The listing builds one solid part. Answer for the finished solid, in the listing's coordinates (mm). Face numbers are marked on the shaded views. A direction names the side the tool comes from. Give positions to 0.01 mm unless a question says otherwise; leave off trailing zeros. Order: outer loops, then holes, each group sorted by start corner. A loop starts at its lowest first (then second) coordinate and runs counter-clockwise, first axis right, second up.
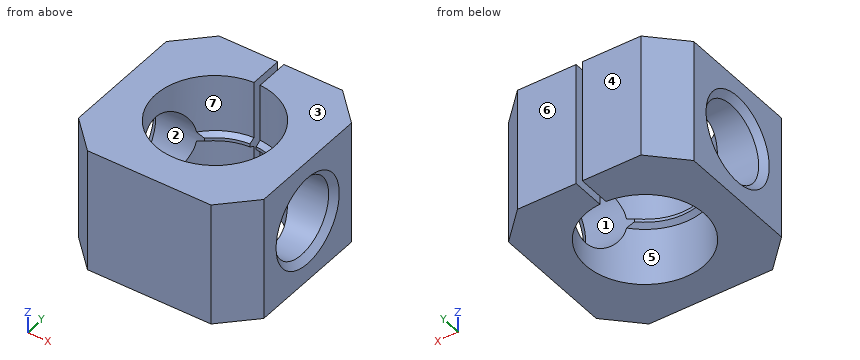
```python
from build123d import *

# Parameters (mm, degrees)
SKETCH047_W     = 30
SKETCH047_H     = 30
SKETCH047_R     = 9.6
PAD018_DEPTH    = 20
SKETCH049_W     = 1
SKETCH049_H     = 15
POCKET028_DEPTH = 20
SKETCH050_R     = 6.2
POCKET029_DEPTH = 40
CHAMFER004_SIZE = 1
CHAMFER005_SIZE = 5


with BuildPart() as part:
    # Sketch047 → Pad018 (new body)
    with BuildSketch(Plane.XY):
        Rectangle(SKETCH047_W, SKETCH047_H)
        Circle(SKETCH047_R, mode=Mode.SUBTRACT)
    extrude(amount=PAD018_DEPTH)

    # Sketch048 → Revolution002 (revolve)
    with BuildSketch(Plane.YZ):
        Polygon((9.6, 10.75), (9.6, 9.25), (8.7, 9.75), (8.7, 10.25), align=None)
    revolve(axis=Axis((0, 0, 0), (0, 0, 1)))

    # Sketch049 (on Face11 of Revolution002) → Pocket028 (cut)
    with BuildSketch(Plane.XY.offset(20)):
        with Locations((0, 7.5)):
            Rectangle(SKETCH049_W, SKETCH049_H)
    extrude(amount=-POCKET028_DEPTH, mode=Mode.SUBTRACT)

    # Sketch050 (on Face12 of Pocket028) → Pocket029 (cut)
    with BuildSketch(Plane(origin=(-15, 0, 0), x_dir=(0, -1, 0), z_dir=(-1, 0, 0))):
        with Locations((0, 10)):
            Circle(SKETCH050_R)
    extrude(amount=-POCKET029_DEPTH, mode=Mode.SUBTRACT)

    # Chamfer004
    chamfer004_edges = [part.edges().sort_by_distance(p)[0] for p in [
        (-15, 6.2, 10),
        (15, 6.2, 10),
    ]]
    chamfer(chamfer004_edges, length=CHAMFER004_SIZE)

    # Chamfer005
    chamfer005_edges = [part.edges().sort_by_distance(p)[0] for p in [
        (-15, -15, 10),
        (-15, 15, 10),
        (15, -15, 10),
        (15, 15, 10),
    ]]
    chamfer(chamfer005_edges, length=CHAMFER005_SIZE)


solid = part.part
```
1) Find section B-B (y = 12.5). Write down the section's boundary in (x, z).
Geometry says:
outline: (-12.5, 0) - (-0.5, 0) - (-0.5, 20) - (-12.5, 20) - close; (0.5, 0) - (12.5, 0) - (12.5, 20) - (0.5, 20) - close
2) Find section D-D (z = 17.75). Write down the section's boundary in (x, y).
Geometry says:
outline: (-15, -10) - (-10, -15) - (10, -15) - (15, -10) - (15, 10) - (10, 15) - (0.5, 15) - (0.5, 9.59) arc R9.6 cw (long way) to (-0.5, 9.59) - (-0.5, 15) - (-10, 15) - (-15, 10) - close
3) Find section A-A (y = 0). Write down the section's boundary in (x, z), then the cut area to 3 significant figures.
Geometry says:
outline: (-15, 0) - (-9.6, 0) - (-9.6, 3.8) - (-14, 3.8) - (-15, 2.8) - close; (-15, 17.2) - (-14, 16.2) - (-9.6, 16.2) - (-9.6, 20) - (-15, 20) - close; (9.6, 0) - (15, 0) - (15, 2.8) - (14, 3.8) - (9.6, 3.8) - close; (9.6, 16.2) - (14, 16.2) - (15, 17.2) - (15, 20) - (9.6, 20) - close
area: 80.1 mm2
4) Straight lines are drawn through the part: probe 1 along Z at (x, y) = (-11.25, 0); probe 2 along Y at (x, z) = (-7.5, 10); probe 3 along Y at (x, z) = (-0.25, 18). For each, find the intervals that lie inside material, in ascending order.
Geometry says:
probe 1: z = 0 to 3.8, 16.2 to 20
probe 2: y = -15 to -6.2, 6.2 to 15
probe 3: y = -15 to -9.6
5) Given P1, Ø8, axis at x = 5.5, y = -0.5, coming from the +Z side, flat-ended and moving along its own axis, determine where the tip first touches the part or whether it passes through.
Geometry says:
P1: passes through
6) For a pull along Y with two mould halves and no side action, classify the marked faces 1, 2, 3 and 4 as +Y half, -Y half, draft (parallel to the pull), parting line (faces both ways), or undercut.
Geometry says:
face 1: undercut
face 2: undercut
face 3: draft
face 4: +Y half
7) Find section C-C (x = 0). Write down the section's boundary in (y, z), then the cut area to 3 significant figures.
Geometry says:
outline: (-15, 0) - (-9.6, 0) - (-9.6, 9.25) - (-8.7, 9.75) - (-8.7, 10.25) - (-9.6, 10.75) - (-9.6, 20) - (-15, 20) - close
area: 109 mm2
8) A tool of negligible diameter and unlimited length cuts with its end or side. For the marked faces 5, 6 and 7, from which of +Z, -Z, +X, -X, +Y, -Y can it reach the whole face along a straight path? Write none if from no direction.
Geometry says:
face 5: -Z
face 6: +Z, -Z, +X, -X, +Y
face 7: +Z
